```python
from build123d import *

# Parameters (mm, degrees)
F0_W     = 5
F0_H     = 66
F0_W_2   = 16.5
F1_DEPTH = 21
F2_DEPTH = 4
F3_W     = 38
F3_H     = 2
F4_DEPTH = 8


# Not quite as in the source:
# - a feature names something its author has since deleted; it is built from what else it names


with BuildPart() as f1:
    # F0 (on Front) → F1 (new body)
    with BuildSketch(Plane.XZ):
        with Locations((-35, -33)):
            Rectangle(F0_W, F0_H)
        with Locations((-45.75, -33)):
            Rectangle(F0_W_2, F0_H)
        with Locations((-24.25, -33)):
            Rectangle(F0_W_2, F0_H)
    extrude(amount=F1_DEPTH)

    # F0 (on Front) → F2 (join)
    with BuildSketch(Plane.XZ):
        with Locations((-35, -33)):
            Rectangle(F0_W, F0_H)
    extrude(amount=-F2_DEPTH)

    # F3 (on face) → F4 (join)
    with BuildSketch(Plane.XZ.offset(21)):
        with Locations((-35, -1)):
            Rectangle(F3_W, F3_H)
    extrude(amount=F4_DEPTH)


solid = f1.part
```
Geometry check sheet. Reference: the model listing, model coordinates, mm. A direction names the side the tool comes from. Give positions to 0.01 mm unless a question says otherwise; leave off trailing zeros. Order: outer loops, then holes, each group sorted by start corner. A loop starts at its lowest first (then second) coordinate and runs counter-clockwise, first axis right, second up. Notation, with made-up numbers: (-23.75, -24.5) - (16.25, -24.5) arc R14 ccw to (16.25, -3.5) - close; hole circle Ø8 at (6, 10.25). An arc over 180 degrees is marked (long way). Write item = value, one per line. Start each with the question number.
1) Section check A-A (z = -57). Enter the section's corners in (x, y).
2) Section check B-B (x = -51). Enter the section's corners in (y, z), then the cut area to 3 significant figures.
3) Scan lines: L1, parallel to Y at x = -43, z = -37.5; L2, parallel to Y at x = -35, z = -31.5; L3, parallel to Z at x = -28, y = -24.5. Record each from-to range of solid material in increasing order.
4) Section check C-C (y = 1). Enter the section's corners in (x, z).
5) Access from +Z, -Z, +X, -X, +Y, -Y to the whole of each face (thin tool, end or side, straight path). Record for faces 1 (the flat face through (-35, 4, -33)), 2 (the flat face through (-37.5, 2, -33)), 3 (the flat face through (-35, -25, -2)), 4 (the flat face through (-24, 0, -33)), 5 (the flat face through (-54, -11, -33)).
6) Gauge pin test, flat ends, axial feed: pin 1 Ø4 at (x, y) = (-24, -4.5) entering from +Z; pin 2 Ø4 at (x, z) = (-33.5, -26.5) entering from -Y; pin 3 Ø3 at (y, z) = (2, -39.5) entering from +X; pin 4 Ø3 at (y, z) = (2.5, -42.5) entering from -X. Record the tip position at first contact, or that the pin passes through.
Geometry check:
q1.outline = (-54, -21) - (-16, -21) - (-16, 0) - (-32.5, 0) - (-32.5, 4) - (-37.5, 4) - (-37.5, 0) - (-54, 0) - close
q2.outline = (-29, -2) - (-21, -2) - (-21, -66) - (0, -66) - (0, 0) - (-29, 0) - close
q2.area = 1,400 mm2
q3.L1 = -21 to 0
q3.L2 = -21 to 4
q3.L3 = -2 to 0
q4.outline = (-37.5, -66) - (-32.5, -66) - (-32.5, 0) - (-37.5, 0) - close
q5.face_1 = +Z, -Z, +X, -X, +Y
q5.face_2 = +Z, -Z, -X, +Y
q5.face_3 = -Z, +X, -X, -Y
q5.face_4 = +Z, -Z, +X, +Y
q5.face_5 = +Z, -Z, -X, +Y, -Y
q6.pin_1 = 0
q6.pin_2 = -21
q6.pin_3 = -32.5
q6.pin_4 = -37.5
